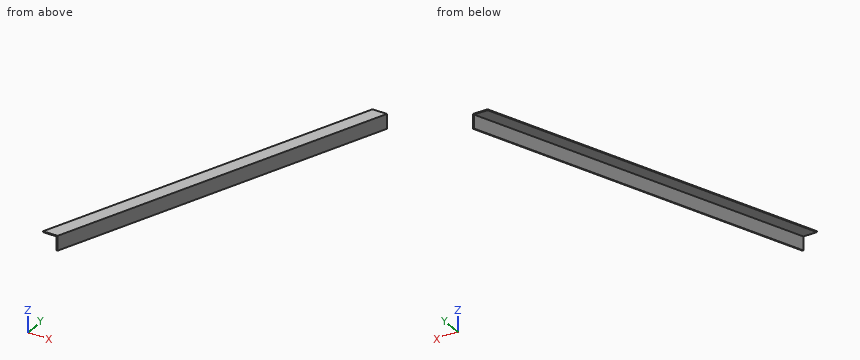
Autodesk Inventor part; units mm, degrees
ref_plane "YZ Plane" through (0, 0, 0) normal (1, 0, 0) x (0, 1, 0)
ref_plane "XZ Plane" through (0, 0, 0) normal (0, 1, 0) x (-1, 0, 0)
ref_plane "XY Plane" through (0, 0, 0) normal (0, 0, 1) x (1, 0, 0)
sketch "Sketch1" plane through (0, 0, 0) normal (1, 0, 0) x (0, 1, 0)
  line L0 (1828.8, -482.6) -> (0, 0)
  line L1 (1828.8, -482.6) -> (1828.8, -533.4)
  line L2 (0, 0) -> (0, -50.8)
  line L3 (0, -50.8) -> (1828.8, -533.4)
  dimension "d3" = 50.8
  dimension "d4" = 50.8
extrude "Extrusion1" add sketch "Sketch1" along normal blind 3.175
sketch "Sketch2" plane through (0, 0, 0) normal (-1, 0, 0) x (0, 0, 1)
  line L0 (0, 0) -> (-482.6, 1828.8)
  line L1 (-482.6, 1828.8) -> (0, 0)
  line L2 (-482.6, 1828.8) -> (-485.775, 1828.8)
  line L3 (-533.4, 1828.8) -> (-482.6, 1828.8)
  line L4 (0, 0) -> (-3.175, 0)
  line L5 (0, 0) -> (-50.8, 0)
  line L6 (-50.8, 0) -> (-533.4, 1828.8)
  line L7 (-3.175, 0) -> (-485.775, 1828.8)
  dimension "d7" = 3.175
  dimension "d8" = 3.175
extrude "Extrusion2" add sketch "Sketch2" along normal blind 47.625 contours L4 L7 L2 L0
properties part number "Front Left Beam"
Read the model definition and answer for the solid it produces. Units are mm, in the model's axes. Coordinates: 2 decimals unless noted, no trailing zeros. Write each loop counter-clockwise with the first axis right and the second up, starting at its lowest first coordinate (ties: lowest second). Pieces come first, ordered by that corner, then holes. Notation, with made-up numbers: (56, 47) -> (85, 47) arc R28 cw to (85, 66) -> close; hole circle Ø3 at (6, 30.25). An arc over 180 degrees is marked (long way). Write item = value, one per line.
(1) Straight lines are drawn through the part: L1, parallel to Z at x = -2, y = 1745.5; L2, parallel to Z at x = -35.5, y = 1282. For each, find the intervals that lie inside material, in ascending order. Write a range as from..to.
From the geometry:
L1 = -463.79..-460.62
L2 = -341.48..-338.31
(2) Section A-A on z = -297 is taken. Write down the section's boundary in (x, y) (3 decimals), plus the area to 3 significant figures.
From the geometry:
outline = (-47.625, 1113.442) -> (0, 1113.442) -> (0, 932.968) -> (3.175, 932.968) -> (3.175, 1125.474) -> (-47.625, 1125.474) -> close
area = 1,180 mm2
(3) Section C-C on x = -15 is taken. Write down the section's boundary in (y, z) (3 decimals).
From the geometry:
outline = (0, -3.175) -> (1828.8, -485.775) -> (1828.8, -482.6) -> (0, 0) -> close
(4) Section B-B on y = 1317 is taken. Write down the section's boundary in (x, z) (3 decimals).
From the geometry:
outline = (-47.625, -350.717) -> (0, -350.717) -> (0, -398.342) -> (3.175, -398.342) -> (3.175, -347.542) -> (-47.625, -347.542) -> close
